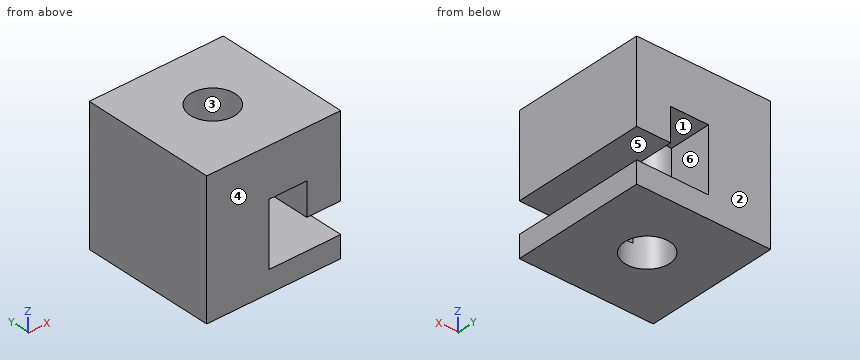
from build123d import *

# Parameters (mm, degrees)
F0_W     = 152.4
F0_H     = 152.4
F1_DEPTH = 152.4
F2_R     = 25.478532
F3_DEPTH = 152.4
F4_W     = 43.219294
F4_H     = 37.589584
F5_DEPTH = 152.4


with BuildPart() as f1:
    # F0 (on Top) → F1 (new body)
    with BuildSketch(Plane.XY):
        Rectangle(F0_W, F0_H)
    extrude(amount=F1_DEPTH)

    # F2 (on face) → F3 (cut)
    with BuildSketch(Plane.XY.offset(152.4)):
        with Locations((0, 2.878058)):
            Circle(F2_R)
    extrude(amount=-F3_DEPTH, mode=Mode.SUBTRACT)

    # F4 (on face) → F5 (cut)
    with BuildSketch(Plane(origin=(0, 76.2, 0), x_dir=(-1, 0, 0), z_dir=(0, 1, 0))):
        with Locations((-16.05138, 78.249803)):
            Rectangle(F4_W, F4_H)
        Polygon((5.558267, 59.455011), (-37.661027, 59.455011), (-76.2, 59.455011), (-76.2, 24.858916), (5.558267, 24.858916), align=None)
    extrude(amount=-F5_DEPTH, mode=Mode.SUBTRACT)


solid = f1.part
Design review of the part built by this model. Coordinates are the model's own, in mm. Face numbers are marked on the shaded views. A direction names the side the tool comes from. Round coordinates to 2 decimals unless told otherwise and drop trailing zeros. Write each loop counter-clockwise with the first axis right and the second up, starting at its lowest first coordinate (ties: lowest second). Pieces come first, ordered by that corner, then holes. Notation, with made-up numbers: (3, 58) -> (57, 58) arc R36 cw to (57, 97) -> close; hole circle Ø3 at (-21, -39.5). An arc over 180 degrees is marked (long way). One line per question, with ' | ' between items.
(1) Take a section at A-A, the plane x = 0. State the section outline as (y, z) points, and give its area (3 significant figures).
Result sheet:
outline: (-76.2, 0) -> (-22.6, 0) -> (-22.6, 24.86) -> (-76.2, 24.86) -> close; (-76.2, 97.04) -> (-22.6, 97.04) -> (-22.6, 152.4) -> (-76.2, 152.4) -> close; (28.36, 0) -> (76.2, 0) -> (76.2, 24.86) -> (28.36, 24.86) -> close; (28.36, 97.04) -> (76.2, 97.04) -> (76.2, 152.4) -> (28.36, 152.4) -> close | area: 8,140 mm2
(2) Take a section at B-B, the plane x = 48.5. State the section outline as (y, z) points.
Result sheet:
outline: (-76.2, 0) -> (76.2, 0) -> (76.2, 24.86) -> (-76.2, 24.86) -> close; (-76.2, 59.46) -> (76.2, 59.46) -> (76.2, 152.4) -> (-76.2, 152.4) -> close
(3) Draft analysis for pull direction Y (two halves, no side actions). For the marked faces 1, 2 and 3, state which applies: released by +Y, released by -Y, zero draft, split by the parting line, or undercut.
Result sheet:
face 1: zero draft | face 2: released by +Y | face 3: undercut
(4) Take a section at C-C, the plane y = -12. State the section outline as (x, z) points, and give its area (3 significant figures).
Result sheet:
outline: (-76.2, 0) -> (-20.68, 0) -> (-20.68, 152.4) -> (-76.2, 152.4) -> close; (20.68, 0) -> (76.2, 0) -> (76.2, 24.86) -> (20.68, 24.86) -> close; (20.68, 97.04) -> (37.66, 97.04) -> (37.66, 59.46) -> (76.2, 59.46) -> (76.2, 152.4) -> (20.68, 152.4) -> close | area: 14,400 mm2
(5) Take a section at D-D, the plane z = 37. State the section outline as (x, y) points.
Result sheet:
outline: (-76.2, -76.2) -> (-5.56, -76.2) -> (-5.56, -21.99) arc R25.48 cw to (-5.56, 27.74) -> (-5.56, 76.2) -> (-76.2, 76.2) -> close
(6) Wall thickness on line 1 (Z direction, x = 27.5, y = 63); line 2 (Z direction, x = 64, y = 63.5); line 3 (X direction, y = -57, z = 89): over which ranges is each line inside the solid? List them lowest first. Write a range as [from, to].
Result sheet:
line 1: [0, 24.86], [97.04, 152.4] | line 2: [0, 24.86], [59.46, 152.4] | line 3: [-76.2, -5.56], [37.66, 76.2]
(7) Machinability: for the marked faces 4, 5 and 6, which of the approach directions +Z, -Z, +X, -X, +Y, -Y give a long, thin tool a straight path to every point of the face, cutting with its end or side? Answer none if there is none.
Result sheet:
face 4: +Z, -Z, +X, -X, -Y | face 5: +X, +Y, -Y | face 6: +Y, -Y
